Can you work these out from the model? Positions are in its coordinate system, mm. A direction names the side the tool comes from. Round coordinates to 2 decimals unless told otherwise and drop trailing zeros.
Q1. Will these pins go through, and if not, where does the flat tip stop? P1, Ø5, axis at x = -347, z = 309, coming from the -Y side; P2, Ø14, axis at y = -13.5, z = 125.5, coming from the -X side; P3, Ø23, axis at y = -16.5, z = 234.5, coming from the +X side.
Q2. If I drill on line 1 (X direction, y = -21, z = 198); line 2 (Z direction, x = -252, y = -6.5); line 3 (X direction, y = -9, z = -170), over which ranges is the centre line in solid material (lowest first)?
Q3. We'd pull the mould along X, two halves only. Please class faces 4 (the face through (434.175, 36.792, -90.466)), 5 (the face through (-257, 16.831, 216)), 6 (the face through (-227.01, -5.77, 233.66)): pulls with the +X half, pulls with the -X half, needs draft (parallel to the pull), parting line crosses it, or undercut.
Q4. For faces 1 (the face through (471.005, -6.408, 122.404)), 2 (the face through (-258.194, -6.408, -274.381)), 3 (the face through (-67.903, 36.792, 453.523)), which set-ups out of +Z, -Z, +X, -X, +Y, -Y let a thin tool reach every point of the face, with its end or its side?
Q5. If we section it at A-A (x = 356.5): Count the separate pieces of the cut face and the enclosed holes in it, plus the area to 3 significant figures.
from build123d import *

# Parameters (mm, degrees)
SWEEP1_START        = -15.278234842
SWEEP1_DEPTH        = 30.556469684
SKETCH6_R           = 13.600984241
SKETCH8_W           = 42.677063854
SKETCH8_H           = 30.556469684
SKETCH9_R           = 15.278234842
BOSS_EXTRUDE1_DEPTH = 131.572
SKETCH10_R          = 15.08646221
BOSS_EXTRUDE2_DEPTH = 162.052
SKETCH11_R          = 15.278234842
BOSS_EXTRUDE3_DEPTH = 296.164
BOSS_EXTRUDE4_REACH = 754.5
BOSS_EXTRUDE5_REACH = 752.76
SKETCH13_W          = 5.310182484
SKETCH13_H          = 30.556469684
SCALE1_SCALE        = 1.5


# Read off the part's stored shape, not the designer's step: Sweep1
with BuildPart() as part:
    # Sweep1 outline → Sweep1 (new body)
    with BuildSketch(Plane(origin=(0, 0, 0), x_dir=(1, 0, 0), z_dir=(0, 1, 0)).offset(SWEEP1_START)):
        with BuildLine():
            Line((-306.148893999, 72.889739207), (-306.148893999, -298.501465503))
            Line((-306.148893999, -298.501465503), (65.123511279, -307.894442395))
            ThreePointArc((65.123511279, -307.894442395), (85.479114327, -304.311825152), (102.843694212, -293.102137949))
            Line((102.843694212, -293.102137949), (305.372800707, -95.632095493))
            ThreePointArc((305.372800707, -95.632095493), (317.018075483, -78.556578014), (321.114366969, -58.2980954))
            Line((321.114366969, -58.2980954), (321.114366969, 313.093109311))
            Line((321.114366969, 313.093109311), (-50.15803831, 322.486086202))
            ThreePointArc((-50.15803831, 322.486086202), (-70.513641359, 318.90346896), (-87.878221243, 307.693781756))
            Line((-87.878221243, 307.693781756), (-290.407327738, 110.2237393))
            ThreePointArc((-290.407327738, 110.2237393), (-302.052602513, 93.148221821), (-306.148893999, 72.889739207))
        make_face()
        with BuildLine():
            Line((-275.592424315, -268.708279376), (-275.592424315, 72.889739207))
            ThreePointArc((-275.592424315, 72.889739207), (-273.896613149, 81.276486376), (-269.075621512, 88.345527557))
            Line((-269.075621512, 88.345527557), (-66.546515017, 285.815570013))
            ThreePointArc((-66.546515017, 285.815570013), (-59.357805776, 290.456234084), (-50.930852017, 291.939390823))
            Line((-50.930852017, 291.939390823), (290.557897284, 283.299923184))
            Line((290.557897284, 283.299923184), (290.557897284, -58.2980954))
            ThreePointArc((290.557897284, -58.2980954), (288.862086118, -66.684842568), (284.041094482, -73.753883749))
            Line((284.041094482, -73.753883749), (81.511987987, -271.223926205))
            ThreePointArc((81.511987987, -271.223926205), (74.323278746, -275.864590277), (65.896324986, -277.347747016))
            Line((65.896324986, -277.347747016), (-275.592424315, -268.708279376))
        make_face(mode=Mode.SUBTRACT)
    extrude(amount=SWEEP1_DEPTH)

    # Sweep2: sweep along a path in Sketch5
    with BuildLine(Plane(origin=(185.347659395, 0, -185.347659395), x_dir=(0.7071067811865562, 0, 0.7071067811865388), z_dir=(-0.7071067811865388, 0, 0.7071067811865562))) as sweep2_path:
        Line((170.396432247, 0), (170.396432247, 41.52665431))
        ThreePointArc((170.396432247, 41.52665431), (153.285610404, 82.835832467), (111.976432247, 99.94665431))
        Line((111.976432247, 99.94665431), (-109.737604983, 99.94665431))
        ThreePointArc((-109.737604983, 99.94665431), (-151.046783139, 82.835832467), (-168.157604983, 41.52665431))
        Line((-168.157604983, 41.52665431), (-168.157604983, 0))
    # Sketch6 → Sweep2 (sweep)
    with BuildSketch(Plane(origin=(0, 0, 0), x_dir=(1, 0, 0), z_dir=(0, 1, 0))):
        with Locations((66.442276603, 304.253042186)):
            Circle(SKETCH6_R)
    sweep2 = sweep(path=sweep2_path.line)

    # Sweep3: sweep along a path in Sketch7
    with BuildLine(Plane(origin=(185.347659395, 0, -185.347659395), x_dir=(0.7071067811865562, 0, 0.7071067811865388), z_dir=(-0.7071067811865388, 0, 0.7071067811865562))) as sweep3_path:
        Line((-168.157604983, 0), (170.396432247, 0))
    # Sketch8 → Sweep3 (sweep)
    with BuildSketch(Plane(origin=(-119.696927762, 0, -122.763491253), x_dir=(0.7159927821962476, 0, -0.6981076821256709), z_dir=(0.6981076821256709, 0, 0.7159927821962476))):
        with Locations((259.973576541, 0)):
            Rectangle(SKETCH8_W, SKETCH8_H)
    sweep3 = sweep(path=sweep3_path.line)

    # Sketch9 → Boss-Extrude1 (add)
    with BuildSketch(Plane(origin=(200.435073348, 0, -200.435073348), x_dir=(-0.7071067811865562, -4.438233130955744e-13, -0.7071067811865388), z_dir=(0.7071067811865388, -4.438233130955853e-13, -0.7071067811865562))):
        with Locations(Location((-2.528524686, 0, 0), (0, 0, 90))):
            Circle(SKETCH9_R)
    extrude(amount=BOSS_EXTRUDE1_DEPTH)

    # Sketch10 → Boss-Extrude2 (add)
    with BuildSketch(Plane(origin=(294.906784072, 0, -294.906784072), x_dir=(0.7071067811865562, 0, 0.7071067811865388), z_dir=(-0.7071067811865388, 0, 0.7071067811865562))):
        with Locations((5.402024194, 0)):
            Circle(SKETCH10_R)
    extrude(amount=-BOSS_EXTRUDE2_DEPTH)

    # Sketch11 → Boss-Extrude3 (add)
    with BuildSketch(Plane(origin=(-174.828459041, 0, 166.200620773), x_dir=(0.6889969243726892, 0, 0.7247642638851441), z_dir=(-0.7247642638851441, 0, 0.6889969243726892))):
        with Locations(Location((5.382894592, 0, 0), (0, 0, 268.068044215))):
            Circle(SKETCH11_R)
    extrude(amount=BOSS_EXTRUDE3_DEPTH)

    # Mirror1: Sweep2, Sweep3 across plane
    add(sweep2.mirror(Plane(origin=(9.771366639, 0, -9.771366639), x_dir=(0.7071067811865562, 0, 0.7071067811865388), z_dir=(-0.7071067811865388, 0, 0.7071067811865562))))
    add(sweep3.mirror(Plane(origin=(9.771366639, 0, -9.771366639), x_dir=(0.7071067811865562, 0, 0.7071067811865388), z_dir=(-0.7071067811865388, 0, 0.7071067811865562))))

    # Sketch12 → Boss-Extrude4 (add, up to next)
    with BuildSketch(Plane(origin=(-122.513234778, 0, -119.452922553), x_dir=(-0.6981076821256531, 1.4154863240378708e-15, 0.715992782196265), z_dir=(-0.715992782196265, 1.4517502346095406e-15, -0.6981076821256531)), mode=Mode.PRIVATE) as boss_extrude4_sk1:
        Polygon((219.277331358, -15.278234842), (219.277331358, 0), (218.737204096, 0), (218.737204096, 15.278234842), (210.99965641, 15.278234842), (210.99965641, -15.278234842), align=None)
    boss_extrude4_tool1 = extrude(boss_extrude4_sk1.sketch, amount=BOSS_EXTRUDE4_REACH, mode=Mode.PRIVATE) - part.part
    add(boss_extrude4_tool1.solids().sort_by_distance((-272.611983, -0.257636, 34.491265))[0])

    # Sketch13 → Boss-Extrude5 (add, up to next)
    with BuildSketch(Plane(origin=(119.869626773, 0, 116.875350401), x_dir=(0.6981076821256531, -1.4154863240378708e-15, -0.715992782196265), z_dir=(0.715992782196265, -1.4517502346095406e-15, 0.6981076821256531)), mode=Mode.PRIVATE) as boss_extrude5_sk1:
        with Locations((-217.936330715, 0)):
            Rectangle(SKETCH13_W, SKETCH13_H)
    boss_extrude5_tool1 = extrude(boss_extrude5_sk1.sketch, amount=BOSS_EXTRUDE5_REACH, mode=Mode.PRIVATE) - part.part
    add(boss_extrude5_tool1.solids().sort_by_distance((-32.2734, 0, 272.91619))[0])


with BuildPart() as part_1:
    # Scale1: scaled about (8.702201295, 12.173569048, -8.333178584)
    add(part.part.scale(SCALE1_SCALE).moved(Location((-4.351100648, -6.086784524, 4.166589292))))


solid = part_1.part
Solution:
1. P1: stops at y = -15.87
1. P2: stops at x = -463.57
1. P3: stops at x = 376.39
2. line 1: x = -463.57 to -417.74, -353.19 to -262.67, 336.38 to 402.03
2. line 2: z = -344.44 to -280.42, 208.67 to 299.19, 411.42 to 457.27
2. line 3: x = -430.9 to -365.25, 332.26 to 422.79, 431.49 to 477.32
3. face 4: parting line crosses it
3. face 5: needs draft
3. face 6: undercut
4. face 1: +Z, +X, +Y, -Y
4. face 2: +Y, -Y
4. face 3: none
5. separate pieces: 5
5. enclosed holes: 0
5. area: 13,400 mm2
